```python
from build123d import *

# Parameters (mm, degrees)
F1_W     = 200
F1_H     = 120
F2_DEPTH = 4
F3_W     = 90
F3_H     = 36
F4_DEPTH = 4
F5_SIZE  = 5
F7_D     = 3.3
F9_D     = 5.5


with BuildPart() as f2:
    # F1 (on Top) → F2 (new body)
    with BuildSketch(Plane.XY):
        with Locations((100, 60)):
            Rectangle(F1_W, F1_H)
    extrude(amount=F2_DEPTH)

    # F3 (on Top) → F4 (cut, through all)
    with BuildSketch(Plane.XY):
        with Locations((100, 60)):
            Rectangle(F3_W, F3_H)
    extrude(amount=F4_DEPTH, mode=Mode.SUBTRACT)

    # F5
    f5_edges = [f2.edges().sort_by_distance(p)[0] for p in [
        (145, 42, 2),
    ]]
    chamfer(f5_edges, length=F5_SIZE)

    # F7 (through all)
    with Locations(Plane(origin=(0, 0, 0), x_dir=(1, 0, 0), z_dir=(0, 0, -1))):
        with Locations((140, -84), (140, -36), (60, -36), (60, -84)):
            Hole(F7_D / 2)

    # F9 (through all)
    with Locations(Plane(origin=(0, 0, 0), x_dir=(1, 0, 0), z_dir=(0, 0, -1))):
        with Locations((25, -110), (25, -60), (25, -10), (175, -110), (175, -60), (175, -10), (10, -110), (10, -60), (10, -10), (190, -110), (190, -60), (190, -10)):
            Hole(F9_D / 2)


solid = f2.part
```
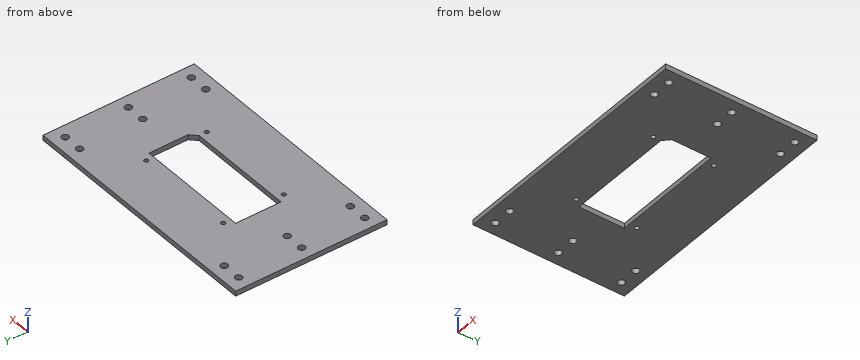
Could you check a few things on this model? Use its own coordinates, in mm. Coordinates: 2 decimals unless noted, no trailing zeros. Order: outer loops, then holes, each group sorted by start corner. A loop starts at its lowest first (then second) coordinate and runs counter-clockwise, first axis right, second up. Notation, with made-up numbers: M 35,-15 L 88,-15 A29 ccw 88,15 Z; hole C 49.25,45 d4. An arc over 180 degrees is marked long. Use a Markdown table: item, result. Add a question column.
Q1. If I drill on L1, parallel to X at y = 110, z = 3.15; L2, parallel to X at y = 60, z = 1.3; L3, parallel to Y at x = 140, z = 2.7, over which ranges is the centre line in solid material (lowest first)?
Q2. I want a section at C-C on x = 190. List the corners of the cut face in (y, z) for me.
Q3. I want a section at A-A on y = 71. List the corners of the cut face in (x, z) for me, then the cut area to 3 significant figures.
Q4. I want a section at B-B on z = 2.35. Give the number of separate pieces and of enclosed holes in the cut face, then the cut area to 3 significant figures.
Q5. I'm going to push a flat-ended pin straight in: pin 1 (5 mm diameter, centred on x = 25, y = 10, fed in from +Z). Where does the tip first touch, or does it pass through?
Q6. I want a section at D-D on y = 110. List the corners of the cut face in (x, z) for me.
Checked values:
| question | item | result |
|---|---|---|
| 1 | L1 | 0 to 7.25, 12.75 to 22.25, 27.75 to 172.25, 177.75 to 187.25, 192.75 to 200 |
| 1 | L2 | 0 to 7.25, 12.75 to 22.25, 27.75 to 55, 145 to 172.25, 177.75 to 187.25, 192.75 to 200 |
| 1 | L3 | 0 to 34.35, 37.65 to 42, 78 to 82.35, 85.65 to 120 |
| 2 | outline | M 0,0 L 7.25,0 L 7.25,4 L 0,4 Z; M 12.75,0 L 57.25,0 L 57.25,4 L 12.75,4 Z; M 62.75,0 L 107.25,0 L 107.25,4 L 62.75,4 Z; M 112.75,0 L 120,0 L 120,4 L 112.75,4 Z |
| 3 | outline | M 0,0 L 55,0 L 55,4 L 0,4 Z; M 145,0 L 200,0 L 200,4 L 145,4 Z |
| 3 | area | 440 mm² |
| 4 | separate pieces | 1 |
| 4 | enclosed holes | 17 |
| 4 | area | 20,500 mm² |
| 5 | pin 1 | through |
| 6 | outline | M 0,0 L 7.25,0 L 7.25,4 L 0,4 Z; M 12.75,0 L 22.25,0 L 22.25,4 L 12.75,4 Z; M 27.75,0 L 172.25,0 L 172.25,4 L 27.75,4 Z; M 177.75,0 L 187.25,0 L 187.25,4 L 177.75,4 Z; M 192.75,0 L 200,0 L 200,4 L 192.75,4 Z |
